Verification items for the finished model (mm, model axes). A direction names the side the tool comes from. Round coordinates to 2 decimals unless told otherwise and drop trailing zeros. Write each loop counter-clockwise with the first axis right and the second up, starting at its lowest first coordinate (ties: lowest second). Pieces come first, ordered by that corner, then holes. Notation, with made-up numbers: M 52.5,-22 L 62.5,-22 A28 cw 62.5,1 Z; hole C 28.5,68 d7. An arc over 180 degrees is marked long. Use a Markdown table: item, result. Add a question column.
from build123d import *

# Parameters (mm, degrees)
SKETCH_1_W          = 104
SKETCH_1_H          = 104
SKETCH_1_W_2        = 92
SKETCH_1_H_2        = 92
EXTRUDE_1_DEPTH     = 7.1
SKETCH_2_W          = 6
SKETCH_2_H          = 40
EXTRUDE_2_DEPTH     = 7
SKETCH_3_W          = 6
SKETCH_3_H          = 8
EXTRUDE_3_DEPTH     = 13
SKETCH_4_W          = 6
SKETCH_4_H          = 40
EXTRUDE_4_DEPTH     = 3
SKETCH_5_W          = 3
SKETCH_5_H          = 14
CUT_EXTRUDE_1_DEPTH = 118.383985279
SKETCH_6_W          = 19
SKETCH_6_H          = 40
SKETCH_6_W_2        = 13
SKETCH_6_H_2        = 24
EXTRUDE_5_DEPTH     = 7
SKETCH_7_W          = 3
SKETCH_7_H          = 4
CUT_EXTRUDE_3_DEPTH = 134.547744271
SKETCH_8_W          = 7.8
SKETCH_8_H          = 6
CUT_EXTRUDE_4_DEPTH = 6
FILLET_START        = 30
FILLET_1_DEPTH      = 40
FILLET_START_2      = -4
FILLET_1_2_DEPTH    = 94
SKETCH_9_W          = 10
SKETCH_9_H          = 10
EXTRUDE_6_DEPTH     = 7.1
SKETCH_10_W         = 122
SKETCH_10_H         = 122
SKETCH_10_W_2       = 112
SKETCH_10_H_2       = 112
EXTRUDE_7_DEPTH     = 7.1
SKETCH_11_R         = 1.5
CUT_EXTRUDE_5_DEPTH = 149.865711297
SKETCH_12_R         = 4
CUT_EXTRUDE_6_DEPTH = 4


with BuildPart() as part:
    # 草图1 → 凸台-拉伸1 (new body)
    with BuildSketch(Plane.XY):
        with Locations((43, 43)):
            Rectangle(SKETCH_1_W, SKETCH_1_H)
        with Locations((43, 43)):
            Rectangle(SKETCH_1_W_2, SKETCH_1_H_2, mode=Mode.SUBTRACT)
    extrude(amount=-EXTRUDE_1_DEPTH)

    # 草图2 → 凸台-拉伸2 (add)
    with BuildSketch(Plane.XY):
        with Locations((92, 50)):
            Rectangle(SKETCH_2_W, SKETCH_2_H)
    extrude(amount=EXTRUDE_2_DEPTH)

    # 草图3 → 凸台-拉伸3 (add)
    with BuildSketch(Plane.XY.offset(7)):
        with Locations((92, 66)):
            Rectangle(SKETCH_3_W, SKETCH_3_H)
        with Locations((92, 34)):
            Rectangle(SKETCH_3_W, SKETCH_3_H)
    extrude(amount=EXTRUDE_3_DEPTH)

    # 草图4 → 凸台-拉伸4 (add)
    with BuildSketch(Plane.XY.offset(20)):
        with Locations((92, 50)):
            Rectangle(SKETCH_4_W, SKETCH_4_H)
    extrude(amount=EXTRUDE_4_DEPTH)

    # 草图5 → 切除-拉伸1 (cut, through all)
    with BuildSketch(Plane.XZ.offset(-30)):
        with Locations((93.5, 16)):
            Rectangle(SKETCH_5_W, SKETCH_5_H)
    extrude(amount=-CUT_EXTRUDE_1_DEPTH, mode=Mode.SUBTRACT)

    # 草图6 → 凸台-拉伸5 (add)
    with BuildSketch(Plane.ZY.offset(-89)):
        with Locations((13.5, 50)):
            Rectangle(SKETCH_6_W, SKETCH_6_H)
        with Locations((13.5, 50)):
            Rectangle(SKETCH_6_W_2, SKETCH_6_H_2, mode=Mode.SUBTRACT)
    extrude(amount=EXTRUDE_5_DEPTH)

    # 草图7 → 切除-拉伸3 (cut, through all)
    with BuildSketch(Plane.ZY.offset(-82)):
        with Locations((13.3, 64)):
            Rectangle(SKETCH_7_W, SKETCH_7_H)
        with Locations((13.3, 36)):
            Rectangle(SKETCH_7_W, SKETCH_7_H)
    extrude(amount=-CUT_EXTRUDE_3_DEPTH, mode=Mode.SUBTRACT)

    # 草图8 → 切除-拉伸4 (cut)
    with BuildSketch(Plane(origin=(92, 0, 0), x_dir=(0, 0, -1), z_dir=(1, 0, 0))):
        with Locations((-12.9, 65)):
            Rectangle(SKETCH_8_W, SKETCH_8_H)
        with Locations((-12.9, 35)):
            Rectangle(SKETCH_8_W, SKETCH_8_H)
    extrude(amount=-CUT_EXTRUDE_4_DEPTH, mode=Mode.SUBTRACT)

    # 圆角1: read off the stored shape, not the designer's step
    # 圆角1 outline → 圆角1 (add)
    with BuildSketch(Plane(origin=(0, 0, 0), x_dir=(1, 0, 0), z_dir=(0, 1, 0)).offset(FILLET_START)):
        with BuildLine():
            ThreePointArc((89, 5.539392014), (87.062257748, -0.376687769), (82, -4))
            Line((82, -4), (89, -4))
            Line((89, -4), (89, 5.539392014))
        make_face()
    extrude(amount=FILLET_1_DEPTH)

    # Fillet 1 2 outline → Fillet 1 2 (add)
    with BuildSketch(Plane(origin=(0, 0, 0), x_dir=(1, 0, 0), z_dir=(0, 1, 0)).offset(FILLET_START_2)):
        with BuildLine():
            Line((89, 0), (89, 5.539392014))
            ThreePointArc((89, 5.539392014), (88.572244047, 2.645926288), (87.325571218, 0))
            Line((87.325571218, 0), (89, 0))
        make_face()
    extrude(amount=FILLET_1_2_DEPTH)

    # 草图9 → 凸台-拉伸6 (add)
    with BuildSketch(Plane(origin=(0, 0, -7.1), x_dir=(-1, 0, 0), z_dir=(0, 0, -1))):
        with Locations((8, -8)):
            Rectangle(SKETCH_9_W, SKETCH_9_H)
        with Locations((-94, -8)):
            Rectangle(SKETCH_9_W, SKETCH_9_H)
        with Locations((8, 94)):
            Rectangle(SKETCH_9_W, SKETCH_9_H)
        with Locations((-94, 94)):
            Rectangle(SKETCH_9_W, SKETCH_9_H)
    extrude(amount=-EXTRUDE_6_DEPTH)

    # 草图10 → 凸台-拉伸7 (add)
    with BuildSketch(Plane(origin=(0, 0, -7.1), x_dir=(-1, 0, 0), z_dir=(0, 0, -1))):
        with Locations((-43, 43)):
            Rectangle(SKETCH_10_W, SKETCH_10_H)
        with Locations((-43, 43)):
            Rectangle(SKETCH_10_W_2, SKETCH_10_H_2, mode=Mode.SUBTRACT)
    extrude(amount=-EXTRUDE_7_DEPTH)

    # 草图11 → 切除-拉伸5 (cut, through all)
    with BuildSketch(Plane.XY):
        with Locations((-11, 97)):
            Circle(SKETCH_11_R)
        with Locations((-11, -11)):
            Circle(SKETCH_11_R)
        with Locations((97, 97)):
            Circle(SKETCH_11_R)
        with Locations((97, -11)):
            Circle(SKETCH_11_R)
    extrude(amount=-CUT_EXTRUDE_5_DEPTH, mode=Mode.SUBTRACT)

    # 草图12 → 切除-拉伸6 (cut)
    with BuildSketch(Plane.XY):
        with Locations((-11, 97)):
            Circle(SKETCH_12_R)
        with Locations((97, 97)):
            Circle(SKETCH_12_R)
        with Locations((-11, -11)):
            Circle(SKETCH_12_R)
        with Locations((97, -11)):
            Circle(SKETCH_12_R)
    extrude(amount=-CUT_EXTRUDE_6_DEPTH, mode=Mode.SUBTRACT)


solid = part.part
1. Scan lines: line 1 along Y through (x, z) = (97, -5.6); line 2 along Y through (x, z) = (97, -1.65). Record each from-to range of solid material in increasing order. Write a range as from..to.
2. Access from +Z, -Z, +X, -X, +Y, -Y to the whole of each face (thin tool, end or side, straight path). Record for faces 1 (the flat face through (-11, -13, -4)), 2 (the flat face through (90, 35, 9)), 3 (the flat face through (82, 50, 5)), 4 (the flat face through (87.1, 62, 8.8)), 5 (the flat face through (42, -9, -4)).
3. Release check for a two-part mould opening along Y. For faces 6 (the flat face through (44, 104, -4)), 7 (the flat face through (86, 33.7, 13)), 8 (the flat face through (88.5, 29.7, 0)) record: +Y half, -Y half, draft (parallel to the pull), parting line (faces both ways), or undercut.
4. Cross-section at A-A on y = 21. Enter the section's corners in (x, z), plus the area to 3 significant figures.
5. Cross-section at B-B on x = 97. Enter the section's corners in (y, z), plus the area to 3 significant figures.
6. Cross-section at D-D on x = 76.5. Enter the section's corners in (y, z), plus the area to 3 significant figures.
7. Depth check by flat-ended pin: pin 1 Ø2.5 at (x, y) = (98, 96) entering from +Z; pin 2 Ø6.5 at (x, y) = (98.5, -10.5) entering from +Z; pin 3 Ø6.5 at (x, z) = (90.5, 13.5) entering from -Y; pin 4 Ø2.5 at (x, y) = (97, 97) entering from -Z. Enter the tip coordinate at first touch or a pass-through.
Answer:
| question | item | result |
|---|---|---|
| 1 | line 1 | y = -18..-12.5, -9.5..-3, 89..95.5, 98.5..104 |
| 1 | line 2 | y = -18..-15, -7..-3, 89..93, 101..104 |
| 2 | face 1 | +Z |
| 2 | face 2 | +X |
| 2 | face 3 | +Z, -Z, -X, +Y, -Y |
| 2 | face 4 | +X, -X |
| 2 | face 5 | +Z, -Z |
| 3 | face 6 | +Y half |
| 3 | face 7 | undercut |
| 3 | face 8 | draft |
| 4 | outline | M -18,-7.1 L -13,-7.1 L -13,0 L -18,0 Z; M -9,-7.1 L -3,-7.1 L -3,0 L -9,0 Z; M 87.33,0 A10 cw 89,-5.54 L 89,-7.1 L 95,-7.1 L 95,0 Z; M 99,-7.1 L 104,-7.1 L 104,0 L 99,0 Z |
| 4 | area | 159 mm^2 |
| 5 | outline | M -18,-7.1 L -12.5,-7.1 L -12.5,-4 L -15,-4 L -15,0 L -18,0 Z; M -9.5,-7.1 L -3,-7.1 L -3,0 L -7,0 L -7,-4 L -9.5,-4 Z; M 89,-7.1 L 95.5,-7.1 L 95.5,-4 L 93,-4 L 93,0 L 89,0 Z; M 98.5,-7.1 L 104,-7.1 L 104,0 L 101,0 L 101,-4 L 98.5,-4 Z |
| 5 | area | 130 mm^2 |
| 6 | outline | M -18,-7.1 L -13,-7.1 L -13,0 L -18,0 Z; M -9,-7.1 L -3,-7.1 L -3,0 L -9,0 Z; M 89,-7.1 L 95,-7.1 L 95,0 L 89,0 Z; M 99,-7.1 L 104,-7.1 L 104,0 L 99,0 Z |
| 6 | area | 156 mm^2 |
| 7 | pin 1 | stops at z = -4 |
| 7 | pin 2 | stops at z = 0 |
| 7 | pin 3 | stops at y = 30 |
| 7 | pin 4 | passes through |
